Can you work these out from the model? Positions are in its coordinate system, mm. A direction names the side the tool comes from. Coordinates: 2 decimals unless noted, no trailing zeros. Order: outer loops, then holes, each group sorted by start corner. A loop starts at its lowest first (then second) coordinate and runs counter-clockwise, first axis right, second up. Notation, with made-up numbers: (-24, -7.75) - (-7, -7.75) arc R30 cw to (-7, 24.25) - close; hole circle Ø10 at (75.5, 63). An arc over 180 degrees is marked (long way). Return JSON: item names as keys, results as strings. Group by question number.
1) Imagine slicing it at C-C (y = 1). Write out the boundary of the cut face in (x, z).
2) Imagine slicing it at A-A (y = 25.5). Write out the boundary of the cut face in (x, z).
3) If we mould it in two halves opening along X, with no side actions, what happens to faces 5 (the face through (-37.5, 0, 1)), 6 (the face through (-24.9, 0, 7)), 7 (the face through (34.11, -24.49, 0.79)), 8 (the face through (-31.89, 26.51, 0.79))? For each: pulls with the +X half, pulls with the -X half, needs draft (parallel to the pull), parting line crosses it, or undercut.
4) Which directions (+Z, -Z, +X, -X, +Y, -Y) give clear straight access to the entire face, cutting with the end or side of a thin tool? Please do faces 1 (the face through (-32.5, 0, 7)), 2 (the face through (-1, -30, 1)), 3 (the face through (-29, 15.3, 7)), 4 (the face through (-29, -15.3, 7)).
5) Imagine slicing it at B-B (x = -30). Write out the boundary of the cut face in (y, z).
6) Imagine slicing it at D-D (z = 9.5). Write out the boundary of the cut face in (x, y).
7) If I drill on line 1 along Y through (x, z) = (33, 0.75); line 2 along Z through (x, y) = (32.5, 7.5); line 3 along X through (y, z) = (10, 6.25), over which ranges is the centre line in solid material (lowest first)?
8) For pin 1 Ø4 at (x, y) = (-33, 25.5) entering from +Z; pin 2 Ø5 at (y, z) = (-6.5, 6) entering from +X; pin 3 Ø4 at (x, z) = (-29, 5) entering from -Y, each with a flat end and sliding along its axis, tell me the tip position at first contact or that it passes through.
```python
from build123d import *

# Parameters (mm, degrees)
F0_W     = 75
F0_H     = 60
F1_DEPTH = 1.6
F2_W     = 7.6
F2_H     = 30.6
F3_DEPTH = 10
F5_D     = 3
F7_D     = 3
F9_D     = 3
F11_D    = 3


with BuildPart() as f1:
    # F0 (on Top) → F1 (new body)
    with BuildSketch(Plane.XY):
        Rectangle(F0_W, F0_H)
    extrude(amount=F1_DEPTH)

    # F2 (on face) → F3 (join)
    with BuildSketch(Plane.XY.offset(1.6)):
        with Locations((-28.7, 2.328e-07)):
            Rectangle(F2_W, F2_H)
    extrude(amount=F3_DEPTH)

    # F5 (through all)
    with Locations(Plane.XY.offset(1.6)):
        with Locations((-33, 25.5)):
            Hole(F5_D / 2)

    # F7 (through all)
    with Locations(Plane(origin=(0, 0, 0), x_dir=(1, 0, 0), z_dir=(0, 0, -1))):
        with Locations((33, -25.5)):
            Hole(F7_D / 2)

    # F9 (through all)
    with Locations(Plane.XY.offset(1.6)):
        with Locations((33, -25.5)):
            Hole(F9_D / 2)

    # F11 (through all)
    with Locations(Plane.XY.offset(1.6)):
        with Locations((-33, -25.5)):
            Hole(F11_D / 2)


with BuildPart() as f12_1:
    # F12: copy of F1
    add(f1.part)


solid = f1.part
```
Calculated:
{
 "1": {"outline": "(-37.5, 0) - (37.5, 0) - (37.5, 1.6) - (-24.9, 1.6) - (-24.9, 11.6) - (-32.5, 11.6) - (-32.5, 1.6) - (-37.5, 1.6) - close"},
 "2": {"outline": "(-37.5, 0) - (-34.5, 0) - (-34.5, 1.6) - (-37.5, 1.6) - close; (-31.5, 0) - (31.5, 0) - (31.5, 1.6) - (-31.5, 1.6) - close; (34.5, 0) - (37.5, 0) - (37.5, 1.6) - (34.5, 1.6) - close"},
 "3": {"face 5": "pulls with the -X half", "face 6": "pulls with the +X half", "face 7": "undercut", "face 8": "undercut"},
 "4": {"face 1": "+Z, -X, +Y, -Y", "face 2": "+Z, -Z, +X, -X, -Y", "face 3": "+Z, +X, -X, +Y", "face 4": "+Z, +X, -X, -Y"},
 "5": {"outline": "(-30, 0) - (30, 0) - (30, 1.6) - (15.3, 1.6) - (15.3, 11.6) - (-15.3, 11.6) - (-15.3, 1.6) - (-30, 1.6) - close"},
 "6": {"outline": "(-32.5, -15.3) - (-24.9, -15.3) - (-24.9, 15.3) - (-32.5, 15.3) - close"},
 "7": {"line 1": "-30 to -27, -24 to 24, 27 to 30", "line 2": "0 to 1.6", "line 3": "-32.5 to -24.9"},
 "8": {"pin 1": "z = 1.6", "pin 2": "x = -24.9", "pin 3": "y = -15.3"}
}
